Source: CAD feature listing. Evaluate the final solid. Frame: model axes, mm. A direction names the side the tool comes from. Round coordinates to 2 decimals unless told otherwise and drop trailing zeros. Order: outer loops, then holes, each group sorted by start corner. A loop starts at its lowest first (then second) coordinate and runs counter-clockwise, first axis right, second up. Notation, with made-up numbers: (47.25, 1.5) - (55.25, 1.5) arc R18 ccw to (55.25, 16.5) - close; hole circle Ø8 at (15.25, 10.25). An arc over 180 degrees is marked (long way). Return JSON: item names as keys, results as strings. Group by question number.
1) Ray query, line 1 (Y direction, x = 0, z = 53); line 2 (Y direction, x = 33, z = 39); line 3 (Y direction, x = 28.5, z = 57.5). Return the intervals inside material, ascending. Write a range as from..to.
2) Access query for faces 4 (the cylindrical face through (-2.994, 22.804, 54.221)), 5 (the cylindrical face through (64.245, -11.923, 52.01)). Directions: +Z, -Z, +X, -X, +Y, -Y. A direction counts if a zero-diameter tool reaches every point of the face in a straight line with its end or side. Return the directions, or none.
3) Contact query for flat-ended pins moving along their axis: P1, Ø3, axis at y = 45.5, z = 92.5, coming from the +X side; P2, Ø4, axis at x = -56.5, z = 48.5, coming from the -Y side; P3, Ø12, axis at x = 36.5, z = 46, coming from the -Y side. Output: stop coordinate, or through.
4) Mould query, pull axis Y, two halves, no side actions, for faces 1 (the cylindrical face through (-44.54, 52.17, 52.01)), 2 (the flat face through (25, 12, 0)), 3 (the conical face through (-17.59, -79.2, 6.13)). Classes: pulls with the +Y half, pulls with the -Y half, needs draft (parallel to the pull), parting line crosses it, or undercut.
5) Section A-A, the plane z = 11. Return loops of the section in (x, y).
Solid Edge part; units mm, degrees
sketch "Sketch1" plane through (0, 0, 0) normal (0, -1, 0) x (1, 0, 0)
  line L0 (0, 0) -> (60, 0)
  line L1 (60, 0) -> (60, 6)
  line L2 (60, 6) -> (83, 6)
  line L3 (83, 6) -> (83, 87.5)
  line L4 (83, 87.5) -> (53, 87.5)
  line L5 (53, 87.5) -> (53, 107)
  line L6 (53, 107) -> (0, 107)
  dimension "D1" = 60
  dimension "D2" = 53
revolve "RevolvedProtrusion1" add sketch "Sketch1" angle 360 about axis through (0, 0, 121.1743) along (0, 0, -1)
hole "Hole_1" at (38, 0, 107) direction (0, 0, -1) diameter 25 depth 70
hole "Hole_2" at (68, 0, 107) direction (0, 0, -1) diameter 25 depth 89.5
pattern_circular "Pattern1" count 6 over 360 about axis through (0, 0, 107) along (0, 0, -1) of "Hole_1"
pattern_circular "Pattern3" count 12 over 360 about axis through (0, 0, 107) along (0, 0, -1) of "Hole_2"
sketch "Sketch2" plane through (0, 0, 107) normal (0, 0, 1) x (1, 0, 0)
  circle A0 centre (0, 0) radius 23
extrude "Cutout1" cut sketch "Sketch2" against normal through all
chamfer "Chamfer_1" distance 2 angle 45 7 edges at (-53, 0, 107) (-23, 0, 107) (-83, 0, 87.5) (-53, 0, 87.5) (-83, 0, 6) (-60, 0, 0) (-23, 0, 0)
properties material "Alluminio, 1060"
Geometry check:
{
 "1": {"line 1": "-83..-80.5, -55.5..-23, 23..55.5, 80.5..83", "line 2": "-76.16..-71.35, -46.43..-11.46, 11.46..46.43, 71.35..76.16", "line 3": "-77.95..-70.11, -47.66..-41.03, -24.78..-8.12, 8.12..24.78, 41.03..47.66, 70.11..77.95"},
 "2": {"face 4": "+Z, -Z", "face 5": "+Z"},
 "3": {"P1": "x = 29.55", "P2": "y = -62.6", "P3": "y = -77.19"},
 "4": {"face 1": "undercut", "face 2": "needs draft", "face 3": "parting line crosses it"},
 "5": {"outline": "circle Ø166 at (0, 0); hole circle Ø46 at (0, 0)"}
}
